Read the model definition and answer for the solid it produces. Units are mm, in the model's axes. Face numbers are marked on the shaded views. A direction names the side the tool comes from. Give positions to 0.01 mm unless a question says otherwise; leave off trailing zeros. Write each loop counter-clockwise with the first axis right and the second up, starting at its lowest first coordinate (ties: lowest second). Pieces come first, ordered by that corner, then holes. Notation, with made-up numbers: (80.5, 11) - (95.5, 11) arc R25 cw to (95.5, 23) - close; hole circle Ø6 at (59, 65). An arc over 180 degrees is marked (long way). Use CSV: the item, a comma, the result in double quotes. Start each with the question number.
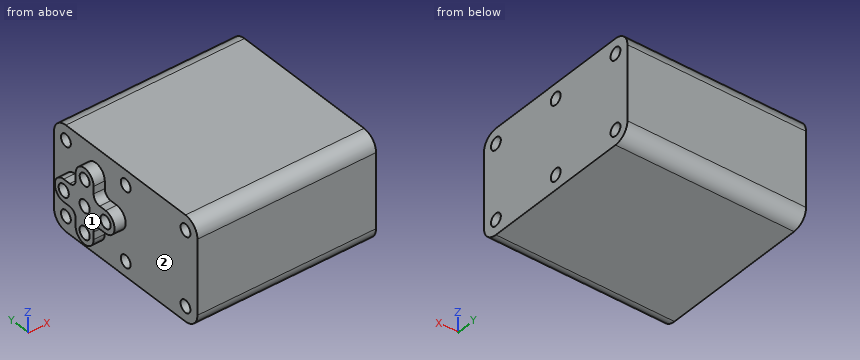
from build123d import *

# Parameters (mm, degrees)
SKETCH_1_R          = 1.7
SKETCH_1_R_2        = 1.65
EXTRUDE_1_DEPTH     = 3
SKETCH_2_W          = 28
SKETCH_2_H          = 48
EXTRUDE_2_DEPTH     = 48
FILLET_1_R          = 4
SKETCH_3_R          = 1.65
CUT_EXTRUDE_1_DEPTH = 4
CUT_EXTRUDE_START   = -4
SKETCH_4_R          = 1.65
CUT_EXTRUDE_2_DEPTH = 4
FILLET_2_R          = 2


with BuildPart() as part:
    # 草图1 → 凸台-拉伸1 (new body)
    with BuildSketch(Plane(origin=(0, 0, 0), x_dir=(0, 0, -1), z_dir=(1, 0, 0))):
        with BuildLine():
            Line((13, -3.07523153), (13, -7.07523153))
            Line((13, -7.07523153), (17, -7.07523153))
            ThreePointArc((17, -7.07523153), (20, -10.07523153), (17, -13.07523153))
            Line((17, -13.07523153), (13, -13.07523153))
            Line((13, -13.07523153), (13, -17.07523153))
            ThreePointArc((13, -17.07523153), (10, -20.07523153), (7, -17.07523153))
            Line((7, -17.07523153), (7, -13.07523153))
            Line((7, -13.07523153), (3, -13.07523153))
            ThreePointArc((3, -13.07523153), (0, -10.07523153), (3, -7.07523153))
            Line((3, -7.07523153), (7, -7.07523153))
            Line((7, -7.07523153), (7, -3.07523153))
            ThreePointArc((7, -3.07523153), (10, -0.07523153), (13, -3.07523153))
        make_face()
        with Locations((10, -3.07523153)):
            Circle(SKETCH_1_R, mode=Mode.SUBTRACT)
        with Locations((3, -10.07523153)):
            Circle(SKETCH_1_R_2, mode=Mode.SUBTRACT)
        with Locations((10, -17.07523153)):
            Circle(SKETCH_1_R, mode=Mode.SUBTRACT)
        with Locations((17, -10.07523153)):
            Circle(SKETCH_1_R, mode=Mode.SUBTRACT)
        with Locations((10, -10.07523153)):
            Circle(SKETCH_1_R, mode=Mode.SUBTRACT)
    extrude(amount=EXTRUDE_1_DEPTH)

    # 草图2 → 凸台-拉伸2 (add)
    with BuildSketch(Plane(origin=(3, 0, 0), x_dir=(0, 0, -1), z_dir=(1, 0, 0))):
        with Locations((10, -20.07523153)):
            Rectangle(SKETCH_2_W, SKETCH_2_H)
    extrude(amount=EXTRUDE_2_DEPTH)

    # 圆角1
    fillet_1_edges = [part.edges().sort_by_distance(p)[0] for p in [
        (27, 3.92476847, -24),
        (27, 3.92476847, 4),
        (27, -44.07523153, 4),
        (27, -44.07523153, -24),
    ]]
    fillet(fillet_1_edges, radius=FILLET_1_R)

    # 草图3 → 切除-拉伸1 (cut)
    with BuildSketch(Plane.ZY.offset(-3)):
        with Locations((-20, -0.07523153)):
            Circle(SKETCH_3_R)
        with Locations((0, -0.07523153)):
            Circle(SKETCH_3_R)
        with Locations((0, -20.07523153)):
            Circle(SKETCH_3_R)
        with Locations((-20, -20.07523153)):
            Circle(SKETCH_3_R)
        with Locations((-20, -40.07523153)):
            Circle(SKETCH_3_R)
        with Locations((0, -40.07523153)):
            Circle(SKETCH_3_R)
    extrude(amount=-CUT_EXTRUDE_1_DEPTH, mode=Mode.SUBTRACT)

    # 草图4 → 切除-拉伸2 (cut)
    with BuildSketch(Plane(origin=(51, 0, 0), x_dir=(0, 0, -1), z_dir=(1, 0, 0)).offset(CUT_EXTRUDE_START)):
        with Locations(Location((0, -0.07523153, 0), (0, 0, 180))):
            Circle(SKETCH_4_R)
        with Locations(Location((20, -0.07523153, 0), (0, 0, 180))):
            Circle(SKETCH_4_R)
        with Locations(Location((0, -20.07523153, 0), (0, 0, 180))):
            Circle(SKETCH_4_R)
        with Locations(Location((20, -20.07523153, 0), (0, 0, 180))):
            Circle(SKETCH_4_R)
        with Locations(Location((0, -40.07523153, 0), (0, 0, 180))):
            Circle(SKETCH_4_R)
        with Locations(Location((20, -40.07523153, 0), (0, 0, 180))):
            Circle(SKETCH_4_R)
    extrude(amount=CUT_EXTRUDE_2_DEPTH, mode=Mode.SUBTRACT)

    # 圆角2
    fillet_2_edges = [part.edges().sort_by_distance(p)[0] for p in [
        (1.5, -13.07523153, -13),
        (1.5, -13.07523153, -7),
        (1.5, -7.07523153, -7),
        (1.5, -7.07523153, -13),
    ]]
    fillet(fillet_2_edges, radius=FILLET_2_R)


solid = part.part
(1) Consider probe 1 along Y at (x, z) = (1.05, -10); probe 2 along Y at (x, z) = (48, -20); probe 3 along Y at (x, z) = (2.3, -3). Determine where each line is inside the solid, lowest interval first.
(2) Which of the six approach directions +Z, -Z, +X, -X, +Y, -Y give full straight-line access (tool end or side, diameter ignored) to the marked faces 1 and 2?
(3) Given P1, Ø5.5, axis at y = -0.08, z = -20, coming from the +X side; P2, Ø2, axis at y = -40.08, z = 0, coming from the +X side; P3, Ø2, axis at y = -40.08, z = -20, coming from the -X side; P4, Ø5, axis at y = -22, z = -4.5, coming from the -X side, each flat-ended and moving along its own axis, determine where each tip first touches the part or whether it passes through.
(4) The part is cut by section A-A on z = -10. Write down the section's boundary in (x, y).
(5) The part is cut by section B-B on y = -27. Write down the section's boundary in (x, z).
Reported:
1,probe 1,"-20.08 to -18.78, -15.38 to -11.78, -8.38 to -4.78, -1.38 to -0.08"
1,probe 2,"-44.08 to -41.73, -38.43 to -21.73, -18.43 to -1.73, 1.57 to 3.92"
1,probe 3,"-13.08 to -11.73, -8.43 to -7.08"
2,face 1,"+Z, -Z, -X, +Y, -Y"
2,face 2,"-X"
3,P1,"x = 51"
3,P2,"x = 47"
3,P3,"x = 7"
3,P4,"x = 3"
4,outline,"(0, -20.08) - (3, -20.08) - (3, -44.08) - (51, -44.08) - (51, 3.92) - (3, 3.92) - (3, -0.08) - (0, -0.08) - (0, -1.38) - (3, -1.38) - (3, -4.78) - (0, -4.78) - (0, -8.38) - (3, -8.38) - (3, -11.78) - (0, -11.78) - (0, -15.38) - (3, -15.38) - (3, -18.78) - (0, -18.78) - close"
5,outline,"(3, -24) - (51, -24) - (51, 4) - (3, 4) - close"
